Model file for the job. Use its own axes, mm. A direction names the side the tool comes from. Coordinates: 2 decimals unless noted, no trailing zeros. Loops run counter-clockwise (first coordinate to the right, second up) from the corner with the lowest first, then second, coordinate; pieces in that order, holes last. Notation, with made-up numbers: (33, 18.25) -> (57, 18.25) arc R28 cw to (57, 48.25) -> close; hole circle Ø11 at (-0.5, 36). An arc over 180 degrees is marked (long way). Use one line per item in the form item = value.
```python
from build123d import *

# Parameters (mm, degrees)
SKETCH_1_R          = 2.6
SKETCH_1_R_2        = 2.5
EXTRUDE_1_DEPTH     = 5
SKETCH_2_R          = 4.5
CUT_EXTRUDE_1_DEPTH = 10
CHAMFER_1_SIZE      = 20
FILLET_1_R          = 10


with BuildPart() as part:
    # 草图1 → 凸台-拉伸1 (new body)
    with BuildSketch(Plane.XY):
        with BuildLine():
            Line((-15, 7.5), (0, 7.5))
            Line((0, 7.5), (15, 7.5))
            Line((15, 7.5), (25, 7.5))
            Line((25, 7.5), (25, 32.5))
            ThreePointArc((25, 32.5), (35, 42.5), (45, 32.5))
            Line((45, 32.5), (45, -7.5))
            ThreePointArc((45, -7.5), (35, -17.5), (25, -7.5))
            Line((25, -7.5), (15, -7.5))
            Line((15, -7.5), (0, -7.5))
            Line((0, -7.5), (-15, -7.5))
            ThreePointArc((-15, -7.5), (-22.5, 0), (-15, 7.5))
        make_face()
        Circle(SKETCH_1_R, mode=Mode.SUBTRACT)
        with Locations((-15, 0)):
            Circle(SKETCH_1_R_2, mode=Mode.SUBTRACT)
    extrude(amount=-EXTRUDE_1_DEPTH)

    # 草图2 → 切除-拉伸1 (cut)
    with BuildSketch(Plane.XY):
        with Locations((35, -7.5)):
            Circle(SKETCH_2_R)
        with Locations((35, 32.5)):
            Circle(SKETCH_2_R)
        with Locations((35, 12.5)):
            Circle(SKETCH_2_R)
    extrude(amount=-CUT_EXTRUDE_1_DEPTH, mode=Mode.SUBTRACT)

    # 倒角1
    chamfer_1_edges = [part.edges().sort_by_distance(p)[0] for p in [
        (25, 7.5, -2.5),
    ]]
    chamfer(chamfer_1_edges, length=CHAMFER_1_SIZE)

    # 圆角1
    fillet_1_edges = [part.edges().sort_by_distance(p)[0] for p in [
        (25, -7.5, -2.5),
    ]]
    fillet(fillet_1_edges, radius=FILLET_1_R)


solid = part.part
```
Q1. Band-saw the part on B-B, the plane y = 12.5. Write the cut outline in (x, z).
Result:
outline = (10, -5) -> (30.5, -5) -> (30.5, 0) -> (10, 0) -> close; (39.5, -5) -> (45, -5) -> (45, 0) -> (39.5, 0) -> close
Q2. Wall check: line 1 along Y through (x, z) = (35, -2.35); line 2 along Y through (x, z) = (-15, -3.8); line 3 along X through (y, z) = (1, -1.7). Give the ranges that are in metal, low to high.
Result:
line_1 = -17.5 to -12, -3 to 8, 17 to 28, 37 to 42.5
line_2 = -7.5 to -2.5, 2.5 to 7.5
line_3 = -22.43 to -17.29, -12.71 to -2.4, 2.4 to 45
Q3. Band-saw the part on D-D, the plane y = 0. Write the cut outline in (x, z).
Result:
outline = (-22.5, -5) -> (-17.5, -5) -> (-17.5, 0) -> (-22.5, 0) -> close; (-12.5, -5) -> (-2.6, -5) -> (-2.6, 0) -> (-12.5, 0) -> close; (2.6, -5) -> (45, -5) -> (45, 0) -> (2.6, 0) -> close
Q4. Which spindle directions (+Z, -Z, +X, -X, +Y, -Y) get a long thin tool onto all of the face, cutting with end or side? Do faces 1 (the face through (-5, 7.5, -2)), 2 (the face through (2, -7.5, -2)), 3 (the face through (39.292, 13.852, -2.465)). Say none if no direction does.
Result:
face_1 = +Z, -Z, -X, +Y
face_2 = +Z, -Z, -X, -Y
face_3 = +Z, -Z
Q5. Band-saw the part on A-A, the plane x = 0. Write the cut outline in (y, z).
Result:
outline = (-7.5, -5) -> (-2.6, -5) -> (-2.6, 0) -> (-7.5, 0) -> close; (2.6, -5) -> (7.5, -5) -> (7.5, 0) -> (2.6, 0) -> close
Q6. Pin check, flat tips, straight feed: pin 1 Ø2.5 at (y, z) = (29.5, -3) entering from -X; pin 2 Ø1.5 at (y, z) = (-9, -4) entering from +X. Stop position of each tip, or through.
Result:
pin_1 = 25
pin_2 = 44.97
Q7. Mould opens along Y. For faces 4 (the face through (19, 6, 0)), 5 (the face through (-0.338, 2.578, -2.465)), 6 (the face through (15.1, 17.6, -2.5)) say: released by +Y, released by -Y, zero draft, split by the parting line, or undercut.
Result:
face_4 = zero draft
face_5 = undercut
face_6 = released by +Y
Q8. Band-saw the part on C-C, the plane x = 35. Write the cut outline in (y, z).
Result:
outline = (-17.5, -5) -> (-12, -5) -> (-12, 0) -> (-17.5, 0) -> close; (-3, -5) -> (8, -5) -> (8, 0) -> (-3, 0) -> close; (17, -5) -> (28, -5) -> (28, 0) -> (17, 0) -> close; (37, -5) -> (42.5, -5) -> (42.5, 0) -> (37, 0) -> close
